```python
from build123d import *

# Parameters (mm, degrees)
SKETCH1_R               = 15.875
BOSS_EXTRUDE1_DEPTH     = 20.701
SWEEP1_PROFILE_R        = 9.525
SWEEP2_PROFILE_R        = 9.525
CUT_EXTRUDE2_REACH      = 369.057
SKETCH36_R              = 7.9375
CUT_EXTRUDE3_REACH      = 369.057
CUT_EXTRUDE3_END_RADIUS = 15.875
SKETCH37_R              = 7.9375
SKETCH77_R              = 15.875
BOSS_EXTRUDE2_DEPTH     = 41.402
CUT_EXTRUDE1_REACH      = 264.618
SKETCH2_R               = 12.7


with BuildPart() as part:
    # Sketch1 → Boss-Extrude1 (new, symmetric)
    with BuildSketch(Plane(origin=(0, 0, 0), x_dir=(1, 0, 0), z_dir=(0, 0.34202014332566943, 0.9396926207859081))):
        with Locations(Location((0, 0, 0), (0, 0, 270))):
            Circle(SKETCH1_R)
    extrude(amount=BOSS_EXTRUDE1_DEPTH, both=True)

    # Sweep1: sweep along a path in Sketch4
    with BuildLine(Plane(origin=(0, 3.019604439, 4.156128957), x_dir=(1, 0, 0), z_dir=(0, 0.5877852522924744, 0.8090169943749467))) as sweep1_path:
        Line((-5.08, -3.732436352), (-132.08, 216.238016209))
    # Sweep1 profile (on start of the path) → Sweep1 (sweep)
    with BuildSketch(Plane(origin=(-5.08, 0, 6.35), x_dir=(0, 0.5877852522924744, 0.8090169943749466), z_dir=(-0.5000000000000013, 0.7006292692220355, -0.5090369604551278))):
        Circle(SWEEP1_PROFILE_R)
    sweep(path=sweep1_path.line)

    # Sweep2: sweep along a path in Sketch15
    with BuildLine(Plane(origin=(0, 3.019604439, 4.156128957), x_dir=(1, 0, 0), z_dir=(0, 0.5877852522924744, 0.8090169943749467))) as sweep2_path:
        Line((5.08, -3.732436352), (132.08, 216.238016209))
    # Sweep2 profile (on start of the path) → Sweep2 (sweep)
    with BuildSketch(Plane(origin=(5.08, 0, 6.35), x_dir=(0, 0.5877852522924744, 0.8090169943749466), z_dir=(0.500000000000001, 0.7006292692220356, -0.5090369604551279))):
        Circle(SWEEP2_PROFILE_R)
    sweep(path=sweep2_path.line)

    # Sketch36 → Cut-Extrude2 (cut, up to next)
    with BuildSketch(Plane(origin=(-126.653807651, 177.474729397, -128.942938553), x_dir=(0.8655546227004349, 0.3849101606410903, -0.32040499895781577), z_dir=(-0.500000000000001, 0.7006292692220356, -0.5090369604551278)), mode=Mode.PRIVATE) as cut_extrude2_sk1:
        with Locations(Location((-6.431589227, -4.927896453, 0), (0, 0, 268.110697529))):
            Circle(SKETCH36_R)
    cut_extrude2_tool1 = extrude(cut_extrude2_sk1.sketch, amount=-CUT_EXTRUDE2_REACH, mode=Mode.PRIVATE) & part.part
    add(cut_extrude2_tool1.solids().sort_by_distance((-132.08, 177.959834, -122.945388))[0], mode=Mode.SUBTRACT)

    # Cut-Extrude3: up to this cylinder (the profile starts outside it)
    cut_extrude3_end = Plane(origin=(0, -18.696540004, -51.368321484), z_dir=(0, -0.34202014332566943, -0.9396926207859081)) * Cylinder(CUT_EXTRUDE3_END_RADIUS, 770.864, mode=Mode.PRIVATE)
    # Sketch37 → Cut-Extrude3 (cut, up to the surface)
    with BuildSketch(Plane(origin=(126.653807651, 177.474729397, -128.942938553), x_dir=(0.865554622700435, -0.3849101606410899, 0.3204049989578159), z_dir=(0.5000000000000008, 0.7006292692220356, -0.5090369604551279)), mode=Mode.PRIVATE) as cut_extrude3_sk1:
        with Locations(Location((6.431589227, -4.927896453, 0), (0, 0, 271.889302471))):
            Circle(SKETCH37_R)
    cut_extrude3_tool1 = extrude(cut_extrude3_sk1.sketch, amount=-CUT_EXTRUDE3_REACH, mode=Mode.PRIVATE) - cut_extrude3_end
    add(cut_extrude3_tool1.solids().sort_by_distance((132.08, 177.959834, -122.945388))[0], mode=Mode.SUBTRACT)

    # Sketch77 → Boss-Extrude2 (add)
    with BuildSketch(Plane(origin=(0, 7.080158987, 19.452576943), x_dir=(1, 0, 0), z_dir=(0, 0.34202014332566943, 0.9396926207859082))):
        with Locations(Location((0, 0, 0), (0, 0, 270))):
            Circle(SKETCH77_R)
    extrude(amount=-BOSS_EXTRUDE2_DEPTH)

    # Sketch2 → Cut-Extrude1 (cut, up to next)
    with BuildSketch(Plane(origin=(0, -7.080158987, -19.452576943), x_dir=(-1, 0, 0), z_dir=(0, -0.34202014332566943, -0.9396926207859081)), mode=Mode.PRIVATE) as cut_extrude1_sk1:
        with Locations(Location((0, 0, 0), (0, 0, 90))):
            Circle(SKETCH2_R)
    cut_extrude1_tool1 = extrude(cut_extrude1_sk1.sketch, amount=-CUT_EXTRUDE1_REACH, mode=Mode.PRIVATE) & part.part
    add(cut_extrude1_tool1.solids().sort_by_distance((0, -7.080159, -19.452577))[0], mode=Mode.SUBTRACT)


solid = part.part
```
Source: CAD feature listing. Evaluate the final solid. Frame: model axes, mm. A direction names the side the tool comes from. Round coordinates to 2 decimals unless told otherwise and drop trailing zeros. Use a Markdown table: item, result. Add a question column.
1. Reachability of faces 1 (the flat face through (-125.32, 179.847, -126.988)), 2 (the cylindrical face through (-12.978, 9.487, -0.666)) from +Z, -Z, +X, -X, +Y, -Y: full face, straight path, thin tool, end or side. Return the list, or none.
2. Mould query, pull axis X, two halves, no side actions, for faces 3 (the cylindrical face through (3.815, 11.284, -4.415)), 4 (the flat face through (138.84, 173.53, -122.4)), 5 (the cylindrical face through (67.21, 91.18, -67.68)), 6 (the flat face through (13.009, 7.15, 19.427)). Classes: pulls with the +X half, pulls with the -X half, needs draft (parallel to the pull), parting line crosses it, or undercut.
3. Contact query for flat-ended pins moving along their axis: P1, Ø12, axis at x = -103, z = -106.5, coming from the +Y side; P2, Ø3, axis at x = 97, z = -82, coming from the -Y side. Output: stop coordinate, or through.
4. Section query A-A on z = -47.5. Give the number of separate pieces and of enclosed holes in the cut face, then the cut area to 3 significant figures.
5. Line query: line 1 (Z direction, x = -38, y = 36); line 2 (Y direction, x = -110, z = -100); line 3 (Y direction, x = 38, z = -31.5). Output: solid intervals per line, ascending.
Reported:
| question | item | result |
|---|---|---|
| 1 | face 1 | -Z, -X, +Y |
| 1 | face 2 | none |
| 2 | face 3 | undercut |
| 2 | face 4 | pulls with the +X half |
| 2 | face 5 | undercut |
| 2 | face 6 | needs draft |
| 3 | P1 | stops at y = 161.99 |
| 3 | P2 | stops at y = 111.15 |
| 4 | separate pieces | 2 |
| 4 | enclosed holes | 2 |
| 4 | area | 342 mm² |
| 5 | line 1 | z = -30.99 to -28.48, -16.1 to -13.59 |
| 5 | line 2 | y = 133.35 to 135.58, 157.81 to 160.03 |
| 5 | line 3 | y = 36.51 to 38.89, 59.44 to 61.82 |
